```python
from build123d import *

# Parameters (mm, degrees)
SKETCH1_R      = 1.45
SKETCH1_R_2    = 1
SKETCH1_R_3    = 1.5
SKETCH1_W      = 22.7
SKETCH1_H      = 12.5
SKETCH1_W_2    = 10
SKETCH1_H_2    = 3.175
SKETCH1_W_3    = 3.175
SKETCH1_H_3    = 7
SKETCH1_W_4    = 28.701572838
SKETCH1_H_4    = 17.835977406
EXTRUDE1_DEPTH = 3.175


with BuildPart() as part:
    # Sketch1 → Extrude1 (new body)
    with BuildSketch(Plane(origin=(0, 0, 0), x_dir=(0, 0, -1), z_dir=(1, 0, 0))):
        Polygon((-106.598842421, -37.036692127), (13.557602199, -37.036692127), (13.557602199, -30.485333973), (3.557602199, -30.485333973), (3.557602199, -27.310333973), (13.557602199, -27.310333973), (13.557602199, -20.211692127), (-18.865609087, -20.211692127), (-18.865609087, 29.788307873), (-32.282953974, 29.936573589), (-32.282953974, 22.936573589), (-35.457953974, 22.936573589), (-35.457953974, 29.936573589), (-38.865609087, 29.788307873), (-106.598842421, 15.913307873), (-106.598842421, 5.913307873), (-96.598842421, 5.913307873), (-96.598842421, 2.738307873), (-106.598842421, 2.738307873), (-106.598842421, -27.261692127), (-96.598842421, -27.261692127), (-96.598842421, -30.436692127), (-106.598842421, -30.436692127), align=None)
        with Locations((-79.418842421, -28.849192127)):
            Circle(SKETCH1_R, mode=Mode.SUBTRACT)
        with Locations((-60.661798953, -21.011692127)):
            Circle(SKETCH1_R_2, mode=Mode.SUBTRACT)
        with Locations((-32.961798953, -21.011692127)):
            Circle(SKETCH1_R_2, mode=Mode.SUBTRACT)
        with Locations((-33.870453974, 13.93657382)):
            Circle(SKETCH1_R, mode=Mode.SUBTRACT)
        with Locations((-74.848842421, 4.325807873)):
            Circle(SKETCH1_R_3, mode=Mode.SUBTRACT)
        with Locations((-46.811798953, -21.011692127)):
            Rectangle(SKETCH1_W, SKETCH1_H, mode=Mode.SUBTRACT)
        with Locations((-11.510665381, -28.849192127)):
            Rectangle(SKETCH1_W_2, SKETCH1_H_2, mode=Mode.SUBTRACT)
        with Locations((-48.098842421, 4.325807873)):
            Rectangle(SKETCH1_W_2, SKETCH1_H_2, mode=Mode.SUBTRACT)
        with Locations((-33.874298953, 1.43657382)):
            Rectangle(SKETCH1_W_3, SKETCH1_H_3, mode=Mode.SUBTRACT)
        with Locations((-83.72320649, -11.157017929)):
            Rectangle(SKETCH1_W_4, SKETCH1_H_4, mode=Mode.SUBTRACT)
    extrude(amount=EXTRUDE1_DEPTH)


solid = part.part
```
Build history of the part. All positions in model axes, mm. A direction names the side the tool comes from. Coordinates: 2 decimals unless noted, no trailing zeros. Order: outer loops, then holes, each group sorted by start corner. A loop starts at its lowest first (then second) coordinate and runs counter-clockwise, first axis right, second up. Notation, with made-up numbers: (84.5, 54) -> (105.5, 54) arc R32 ccw to (105.5, 82) -> close; hole circle Ø9 at (66.5, 25.5). An arc over 180 degrees is marked (long way). Answer in a Markdown table with one row per item. Add a question column.
Q1. Band-saw the part on D-D, the plane y = 17.5. List the corners of the cut face in (x, z) (3 decimals), then the cut area to 3 significant figures.
Q2. Band-saw the part on C-C, the plane x = 1.6. Give the number of separate pieces and of enclosed holes in the cut face, then the cut area to 3 significant figures.
Q3. Drop flat-ended pins along their axis: pin 1 (1 mm diameter, centred on x = 2.5, y = -29.5, fed in from -Z); pin 2 (1 mm diameter, centred on x = 1.5, z = 101, fed in from +Y); pin 3 (1 mm diameter, centred on x = 2, y = 2.5, fed in from -Z); pin 4 (1.7 mm diameter, centred on y = -28.85, z = 79.42, fed in from -X). Give the stop position or say it passes through.
Q4. Which spindle directions (+Z, -Z, +X, -X, +Y, -Y) get a long thin tool onto all of the face, cutting with end or side? Do faces 4 (the face through (2, -20.212, 2)), 5 (the face through (2, 5.913, 102)), 6 (the face through (2, -34, 106.599)), 7 (the face through (2, 26, 35.458)), 8 (the face through (2, 2.738, 48)). Say none if no direction does.
Q5. Band-saw the part on A-A, the plane z = -6. List the corners of the cut face in (x, y) (3 decimals).
Q6. Mould opens along Z. For faces 1 (the face through (2, 26, 32.283)), 2 (the face through (2, -29, -3.558)), 3 (the face through (2, -12, 106.599)) say: +Z half, -Z half, draft (parallel to the pull), parting line (faces both ways), or undercut.
Q7. Wall check: line 1 along Z through (x, y) = (2.15, -17.5); line 2 along Y through (x, z) = (0.35, 79.5) (3 decimals); line 3 along Y through (x, z) = (0.8, 36). Give the ranges that are in metal, low to high. Write a range as [from, to].
Q8. Band-saw the part on B-B, the plane y = 24.5. List the corners of the cut face in (x, z) (3 decimals).
Answers follow:
| question | item | result |
|---|---|---|
| 1 | outline | (0, 18.866) -> (3.175, 18.866) -> (3.175, 98.853) -> (0, 98.853) -> close |
| 1 | area | 254 mm^2 |
| 2 | separate pieces | 1 |
| 2 | enclosed holes | 10 |
| 2 | area | 4,910 mm^2 |
| 3 | pin 1 | z = -3.56 |
| 3 | pin 2 | y = 17.16 |
| 3 | pin 3 | z = 18.87 |
| 3 | pin 4 | through |
| 4 | face 4 | -Z, +X, -X, +Y |
| 4 | face 5 | +Z, +X, -X |
| 4 | face 6 | +Z, +X, -X, +Y, -Y |
| 4 | face 7 | +X, -X, +Y |
| 4 | face 8 | +X, -X |
| 5 | outline | (0, -37.037) -> (3.175, -37.037) -> (3.175, -30.485) -> (0, -30.485) -> close; (0, -27.31) -> (3.175, -27.31) -> (3.175, -20.212) -> (0, -20.212) -> close |
| 6 | face 1 | undercut |
| 6 | face 2 | -Z half |
| 6 | face 3 | +Z half |
| 7 | line 1 | [18.87, 35.46], [58.16, 69.37], [98.07, 106.6] |
| 7 | line 2 | [-37.037, -30.297], [-27.401, -20.075], [-2.239, 21.464] |
| 7 | line 3 | [-37.04, -27.26], [-14.76, 29.91] |
| 8 | outline | (0, 18.866) -> (3.175, 18.866) -> (3.175, 32.283) -> (0, 32.283) -> close; (0, 35.458) -> (3.175, 35.458) -> (3.175, 64.681) -> (0, 64.681) -> close |
